from build123d import *

# Parameters (mm, degrees)
SKETCH1_W           = 52
SKETCH1_H           = 23
BOSS_EXTRUDE1_DEPTH = 5
BOSS_EXTRUDE2_DEPTH = 2


with BuildPart() as part:
    # Sketch1 → Boss-Extrude1 (new body)
    with BuildSketch(Plane(origin=(0, 0, 0), x_dir=(1, 0, 0), z_dir=(0, 1, 0))):
        with Locations((26, 11.5)):
            Rectangle(SKETCH1_W, SKETCH1_H)
    extrude(amount=BOSS_EXTRUDE1_DEPTH)

    # Sketch2 → Boss-Extrude2 (add)
    with BuildSketch(Plane(origin=(0, 5, 0), x_dir=(1, 0, 0), z_dir=(0, 1, 0))):
        Polygon((47, 5), (37.5, 5), (37.5, 19), (35.5, 19), (35.5, 3), (49, 3), (49, 19), (47, 19), align=None)
        Polygon((4, 19), (4, 3), (17.5, 3), (17.5, 19), (15.5, 19), (15.5, 5), (6, 5), (6, 19), align=None)
    extrude(amount=BOSS_EXTRUDE2_DEPTH)


solid = part.part
Part model, mm, in its own coordinate system. A direction names the side the tool comes from. Coordinates: 2 decimals unless noted, no trailing zeros. Order: outer loops, then holes, each group sorted by start corner. A loop starts at its lowest first (then second) coordinate and runs counter-clockwise, first axis right, second up.
(1) Probe L1, parallel to X at y = 6.25, z = -16.75; L2, parallel to Y at x = 6, z = -0.75; L3, parallel to Z at x = 48.5, y = 6.25. List the from-to ranges inside material, lowest first.
Check sheet entries:
L1: x = 4 to 6, 15.5 to 17.5, 35.5 to 37.5, 47 to 49
L2: y = 0 to 5
L3: z = -19 to -3
(2) Tool access for faces 4 (the face through (49, 6, -11)), 5 (the face through (4, 6, -11)), 6 (the face through (35.5, 6, -11)), 7 (the face through (37, 6, -19)), 8 (the face through (47, 6, -12)): list every direction of +Z, -Z, +X, -X, +Y, -Y with a clear straight run to the whole face (end or side of a thin tool).
Check sheet entries:
face 4: +Z, -Z, +X, +Y
face 5: +Z, -Z, -X, +Y
face 6: +Z, -Z, +Y
face 7: -Z, +X, -X, +Y
face 8: -Z, +Y
(3) Pin check, flat tips, straight feed: pin 1 Ø1 at (x, y) = (48.5, 6.5) entering from -Z; pin 2 Ø0.6 at (y, z) = (5.5, -10) entering from -X; pin 3 Ø1 at (y, z) = (6, -14) entering from +X. Stop position of each tip, or through.
Check sheet entries:
pin 1: stops at z = -19
pin 2: stops at x = 4
pin 3: stops at x = 49
(4) Slice it at C-C, the plane x = 12. Write the cut outline in (y, z).
Check sheet entries:
outline: (0, -23) - (5, -23) - (5, -5) - (7, -5) - (7, -3) - (5, -3) - (5, 0) - (0, 0) - close
(5) Pull direction X, two halves, no side cores. Call faces 1 (the face through (37.5, 6, -12)), 2 (the face through (5.7, 7, -9.3)), 3 (the face through (52, 2, -11)): pulls with the +X half, pulls with the -X half, needs draft (parallel to the pull), parting line crosses it, or undercut.
Check sheet entries:
face 1: undercut
face 2: needs draft
face 3: pulls with the +X half
(6) Slice it at D-D, the plane x = 27. Write the cut outline in (y, z), and give its area (3 significant figures).
Check sheet entries:
outline: (0, -23) - (5, -23) - (5, 0) - (0, 0) - close
area: 115 mm2
(7) Slice it at A-A, the plane y = 5.75. Write the cut outline in (x, z).
Check sheet entries:
outline: (4, -19) - (6, -19) - (6, -5) - (15.5, -5) - (15.5, -19) - (17.5, -19) - (17.5, -3) - (4, -3) - close; (35.5, -19) - (37.5, -19) - (37.5, -5) - (47, -5) - (47, -19) - (49, -19) - (49, -3) - (35.5, -3) - close
(8) Slice it at B-B, the plane z = -12. Write the cut outline in (x, y).
Check sheet entries:
outline: (0, 0) - (52, 0) - (52, 5) - (49, 5) - (49, 7) - (47, 7) - (47, 5) - (37.5, 5) - (37.5, 7) - (35.5, 7) - (35.5, 5) - (17.5, 5) - (17.5, 7) - (15.5, 7) - (15.5, 5) - (6, 5) - (6, 7) - (4, 7) - (4, 5) - (0, 5) - close
